The drawing under review shows one solid part. Ordinate dimensions are in mm from its lowest x, y, z. Round coordinates to 2 decimals unless told otherwise and drop trailing zeros. Write each loop counter-clockwise with the first axis right and the second up, starting at its lowest first coordinate (ties: lowest second). Pieces come first, ordered by that corner, then holes. Notation, with made-up numbers: (66.5, -33) -> (93.5, -33) arc R15 cw to (93.5, -22) -> close; hole circle Ø11 at (77.5, 60.25). An arc over 180 degrees is marked (long way). Write item = value, one per line. Start each with the question number.
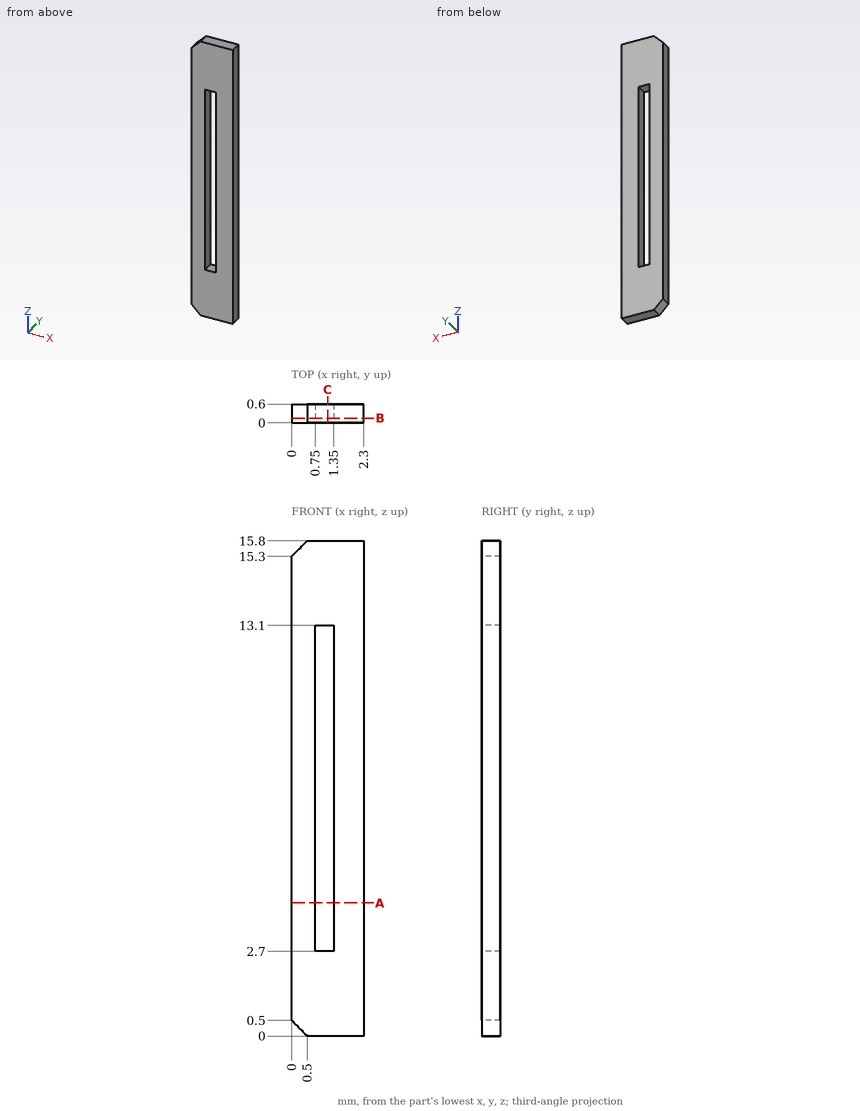
1. Consider section C-C, the plane x = 1.15. Give the boundary of the cut face in (y, z), then the cut area to 3 significant figures.
2. Wall thickness on L1, parallel to X at y = 0.4, z = 3.5; L2, parallel to Z at x = 1.05, y = 0.25; L3, parallel to Z at x = 0.45, y = 0.55: over which ranges is each line inside the solid? List them lowest first. Write a range as from..to.
3. Consider section B-B, the plane y = 0.15. Give the boundary of the cut face in (x, z).
4. Consider section A-A, the plane z = 4.25. Give the boundary of the cut face in (x, y), then the cut area to 3 significant figures.
Outcome:
q1.outline = (0, 0) -> (0.6, 0) -> (0.6, 2.7) -> (0, 2.7) -> close; (0, 13.1) -> (0.6, 13.1) -> (0.6, 15.8) -> (0, 15.8) -> close
q1.area = 3.24 mm2
q2.L1 = 0..0.75, 1.35..2.3
q2.L2 = 0..2.7, 13.1..15.8
q2.L3 = 0.05..15.75
q3.outline = (0, 0.5) -> (0.5, 0) -> (2.3, 0) -> (2.3, 15.8) -> (0.5, 15.8) -> (0, 15.3) -> close; hole (0.75, 2.7) -> (1.35, 2.7) -> (1.35, 13.1) -> (0.75, 13.1) -> close
q4.outline = (0, 0) -> (0.75, 0) -> (0.75, 0.6) -> (0, 0.6) -> close; (1.35, 0) -> (2.3, 0) -> (2.3, 0.6) -> (1.35, 0.6) -> close
q4.area = 1.02 mm2
